Read the model definition and answer for the solid it produces. Units are mm, in the model's axes. Face numbers are marked on the shaded views. A direction names the side the tool comes from. Round coordinates to 2 decimals unless told otherwise and drop trailing zeros. Order: outer loops, then holes, each group sorted by start corner. A loop starts at its lowest first (then second) coordinate and runs counter-clockwise, first axis right, second up. Notation, with made-up numbers: (44, -18.75) -> (76, -18.75) arc R23 ccw to (76, 8.25) -> close; hole circle Ø5 at (3.25, -31). An arc over 180 degrees is marked (long way). One line per item, written item: value. Start each with the question number.
1. Section B-B (y = -4.5) is taken. Give the vertices of the cut face in (x, z).
2. For the marked faces 1 and 2, determine the directions among +Z, -Z, +X, -X, +Y, -Y from which every point of the face is accessible in a straight line to the end or side of a thin tool.
3. Section A-A (z = -2) is taken. Give the vertices of the cut face in (x, y), then the cut area to 3 significant figures.
4. Section D-D (z = 11) is taken. Give the vertices of the cut face in (x, y).
5. Consider line 1 (Z direction, x = -6.8, y = 0); line 2 (X direction, y = -2.75, z = 13). Determine where each line is inside the solid, lowest interval first.
6. Section C-C (x = -5.5) is taken. Give the vertices of the cut face in (y, z), then the cut area to 3 significant figures.
7. The mould has two halves that part along Y. Classify the marked faces 3, 4 and 5: released by +Y, released by -Y, zero draft, split by the parting line, or undercut.
from build123d import *

# Parameters (mm, degrees)
F1_DEPTH = 20
F3_DEPTH = 25


with BuildPart() as f1:
    # F0 (on Top) → F1 (new body)
    with BuildSketch(Plane.XY):
        with BuildLine():
            ThreePointArc((-8, -5), (-7.12132, -7.12132), (-5, -8))
            Line((-5, -8), (5, -8))
            ThreePointArc((5, -8), (7.12132, -7.12132), (8, -5))
            Line((8, -5), (8, 5))
            ThreePointArc((8, 5), (7.12132, 7.12132), (5, 8))
            Line((5, 8), (-5, 8))
            ThreePointArc((-5, 8), (-7.12132, 7.12132), (-8, 5))
            Line((-8, 5), (-8, -5))
        make_face()
        with BuildLine():
            Line((3.5, -6.5), (-3.5, -6.5))
            ThreePointArc((-3.5, -6.5), (-5.62132, -5.62132), (-6.5, -3.5))
            Line((-6.5, -3.5), (-6.5, 3.5))
            ThreePointArc((-6.5, 3.5), (-5.62132, 5.62132), (-3.5, 6.5))
            Line((-3.5, 6.5), (3.5, 6.5))
            ThreePointArc((3.5, 6.5), (5.62132, 5.62132), (6.5, 3.5))
            Line((6.5, 3.5), (6.5, -3.5))
            ThreePointArc((6.5, -3.5), (5.62132, -5.62132), (3.5, -6.5))
        make_face(mode=Mode.SUBTRACT)
    extrude(amount=F1_DEPTH)

    # F2 (on face) → F3 (cut)
    with BuildSketch(Plane.YZ.offset(8)):
        with BuildLine():
            ThreePointArc((1.5, 10), (-1.06066, 11.06066), (0, 8.5))
            ThreePointArc((0, 8.5), (1.06066, 8.93934), (1.5, 10))
        make_face()
    extrude(amount=-F3_DEPTH, mode=Mode.SUBTRACT)

    # F4: F1 across plane


with BuildPart() as f1_1:
    add(f1.part)
    add(f1.part.mirror(Plane.XY))


solid = f1_1.part
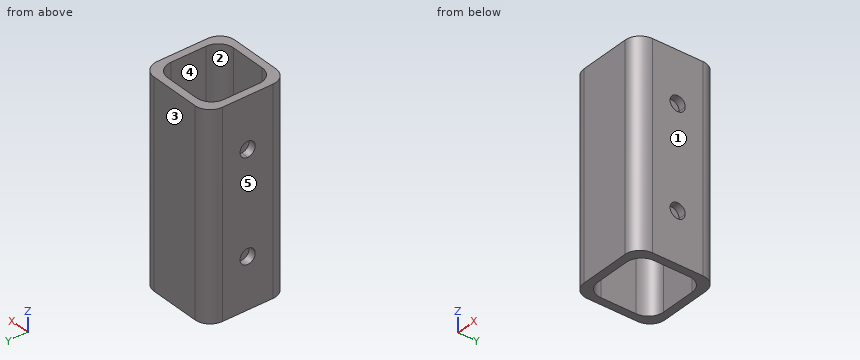
Answer:
1. outline: (-8, -20) -> (-6.33, -20) -> (-6.33, 20) -> (-8, 20) -> close; (6.33, -20) -> (8, -20) -> (8, 20) -> (6.33, 20) -> close
2. face 1: +Z, -Z, +X, +Y, -Y
2. face 2: +Z, -Z
3. outline: (-8, -5) arc R3 ccw to (-5, -8) -> (5, -8) arc R3 ccw to (8, -5) -> (8, 5) arc R3 ccw to (5, 8) -> (-5, 8) arc R3 ccw to (-8, 5) -> close; hole (-6.5, -3.5) arc R3 ccw to (-3.5, -6.5) -> (3.5, -6.5) arc R3 ccw to (6.5, -3.5) -> (6.5, 3.5) arc R3 ccw to (3.5, 6.5) -> (-3.5, 6.5) arc R3 ccw to (-6.5, 3.5) -> close
3. area: 87.0 mm^2
4. outline: (-8, -5) arc R3 ccw to (-5, -8) -> (5, -8) arc R3 ccw to (8, -5) -> (8, -1.12) -> (6.5, -1.12) -> (6.5, -3.5) arc R3 cw to (3.5, -6.5) -> (-3.5, -6.5) arc R3 cw to (-6.5, -3.5) -> (-6.5, -1.12) -> (-8, -1.12) -> close; (-8, 1.12) -> (-6.5, 1.12) -> (-6.5, 3.5) arc R3 cw to (-3.5, 6.5) -> (3.5, 6.5) arc R3 cw to (6.5, 3.5) -> (6.5, 1.12) -> (8, 1.12) -> (8, 5) arc R3 ccw to (5, 8) -> (-5, 8) arc R3 ccw to (-8, 5) -> close
5. line 1: -20 to -11.5, -8.5 to 8.5, 11.5 to 20
5. line 2: -8 to -6.5, 6.5 to 8
6. outline: (-7.96, -20) -> (-5.74, -20) -> (-5.74, 20) -> (-7.96, 20) -> close; (5.74, -20) -> (7.96, -20) -> (7.96, 20) -> (5.74, 20) -> close
6. area: 178 mm^2
7. face 3: released by +Y
7. face 4: undercut
7. face 5: zero draft
